```python
from build123d import *

# Parameters (mm, degrees)
SKETCH1_R           = 5.715
BOSS_EXTRUDE1_DEPTH = 19.05
SKETCH2_R           = 9.525
BOSS_EXTRUDE2_DEPTH = 53.975
SKETCH3_R           = 9.525
BOSS_EXTRUDE3_DEPTH = 53.975


with BuildPart() as part:
    # Sketch1 → Boss-Extrude1 (new body)
    with BuildSketch(Plane(origin=(0, 0, 0), x_dir=(1, 0, 0), z_dir=(0, 1, 0))):
        Circle(SKETCH1_R)
    extrude(amount=BOSS_EXTRUDE1_DEPTH)

    # Sketch2 → Boss-Extrude2 (add)
    with BuildSketch(Plane(origin=(0, 19.05, 0), x_dir=(1, 0, 0), z_dir=(0, 1, 0))):
        Circle(SKETCH2_R)
    extrude(amount=BOSS_EXTRUDE2_DEPTH)

    # Sketch3 → Boss-Extrude3 (add)
    with BuildSketch(Plane.XZ):
        Circle(SKETCH3_R)
    extrude(amount=BOSS_EXTRUDE3_DEPTH)


solid = part.part
```
Geometry: final body of the model. Coordinates: model frame, mm. A direction names the side the tool comes from. Coordinates: 2 decimals unless noted, no trailing zeros. Order: outer loops, then holes, each group sorted by start corner. A loop starts at its lowest first (then second) coordinate and runs counter-clockwise, first axis right, second up. Notation, with made-up numbers: M 39,58 L 78,58 A22 cw 78,92 Z; hole C 58,-24.75 d10. An arc over 180 degrees is marked long. Answer as CSV lines item,"result".
Q1. Line query: probe 1 along Y at (x, z) = (-7, 3.75) (3 decimals); probe 2 along X at (y, z) = (-42.5, -0.25); probe 3 along Z at (x, y) = (-0.5, -28.5). Output: solid intervals per line, ascending. Write a range as [from, to].
Answers:
probe 1,"y = [-53.975, 0], [19.05, 73.025]"
probe 2,"x = [-9.52, 9.52]"
probe 3,"z = [-9.51, 9.51]"
Q2. Section C-C on x = 0. Return the cut outline in (y, z) (3 decimals).
Answers:
outline,"M -53.975,-9.525 L 0,-9.525 L 0,-5.715 L 19.05,-5.715 L 19.05,-9.525 L 73.025,-9.525 L 73.025,9.525 L 19.05,9.525 L 19.05,5.715 L 0,5.715 L 0,9.525 L -53.975,9.525 Z"
Q3. Draft query along Y for faces 1 (the flat face through (0, 0, -6)), 2 (the cylindrical face through (-7.559, -26.61, -5.796)), 3 (the flat face through (0, 73.025, 0)). Return one class per face: pulls with the +Y half, pulls with the -Y half, needs draft (parallel to the pull), parting line crosses it, or undercut.
Answers:
face 1,"undercut"
face 2,"needs draft"
face 3,"pulls with the +Y half"
Q4. Section B-B on z = 0. Return the cut outline in (x, y) (3 decimals), and give its area (3 significant figures).
Answers:
outline,"M -9.525,-53.975 L 9.525,-53.975 L 9.525,0 L 5.715,0 L 5.715,19.05 L 9.525,19.05 L 9.525,73.025 L -9.525,73.025 L -9.525,19.05 L -5.715,19.05 L -5.715,0 L -9.525,0 Z"
area,"2,270 mm^2"
Q5. Section A-A on x = 7.25. Return the cut outline in (y, z) (3 decimals), and give its area (3 significant figures).
Answers:
outline,"M -53.975,-6.178 L 0,-6.178 L 0,6.178 L -53.975,6.178 Z; M 19.05,-6.178 L 73.025,-6.178 L 73.025,6.178 L 19.05,6.178 Z"
area,"1,330 mm^2"
Q6. Set-up query: faces 4 (the flat face through (0, 19.05, 6)), 5 (the cylindrical face through (-7.559, 45.66, 5.796)). Return all of +Z, -Z, +X, -X, +Y, -Y with unobstructed straight access to the full face (end or side cutting, diameter ignored); none if empty.
Answers:
face 4,"none"
face 5,"+Y, -Y"
Q7. First-contact query: P1, Ø3, axis at x = -6.5, z = -7.5, coming from the -Y side (3 decimals); P2, Ø1, axis at x = -7, y = 35, coming from the +Z side; P3, Ø2, axis at y = 20.5, z = 1.5, coming from the +X side; P4, Ø4, axis at y = -30.5, z = -4, coming from the +X side. Flat tips, straight axial feed; report the tip coordinate or a pass-through.
Answers:
P1,"stops at y = -53.975"
P2,"stops at z = 6.96"
P3,"stops at x = 9.51"
P4,"stops at x = 9.31"
Q8. Section D-D on z = -7.75. Return the cut outline in (x, y) (3 decimals).
Answers:
outline,"M -5.537,-53.975 L 5.537,-53.975 L 5.537,0 L -5.537,0 Z; M -5.537,19.05 L 5.537,19.05 L 5.537,73.025 L -5.537,73.025 Z"
